Design review of the part shown in the three views and the two pictorial views. Dimensions are in mm from the part's minimum x, y and z. A direction names the side the tool comes from. Coordinates: 2 decimals unless noted, no trailing zeros. Loops run counter-clockwise (first coordinate to the right, second up) from the corner with the lowest first, then second, coordinate; pieces in that order, holes last. Notation, with made-up numbers: M -17,61 L 4,61 A20 ccw 4,75 Z; hole C 43,-27.75 d11. An arc over 180 degrees is marked long. Answer as a JSON object with one key per item and string values. Group by question number.
Item 1: Tool access review of the marked faces 5, 6 and 7: name each direction out of +Z, -Z, +X, -X, +Y, -Y from which nothing blocks a thin tool from reaching the whole face with its end or side.
Item 2: Wall thickness on L1, parallel to Z at x = 24.5, y = 20; L2, parallel to X at y = 10, z = 2.5: over which ranges is each line inside the solid? List them lowest first. Write a range as from..to.
Item 3: Insertion check: pin 1 (4 mm diameter, centred on x = 47.5, z = 11.5, fed in from -Y); pin 2 (7.5 mm diameter, centred on y = 17, z = 30.5, fed in from +X); pin 3 (2 mm diameter, centred on x = 39.5, y = 18, fed in from +Z). Each pin has a flat end and moves straight along its axis. Give the tip position at first contact, or say it passes through.
Item 4: Add section C-C (y = 10.5). State the section outline as (x, z) points, then the cut area to 3 significant figures.
Item 5: Mouldability with a two-part tool opening along Y and no side actions: class the marked faces 1, 2, 3 and 4 as +Y half, -Y half, draft (parallel to the pull), parting line (faces both ways), or undercut.
Item 6: Add section B-B (x = 9.5). State the section outline as (y, z) points.
Item 7: Add section A-A (z = 5). State the section outline as (x, y) points.
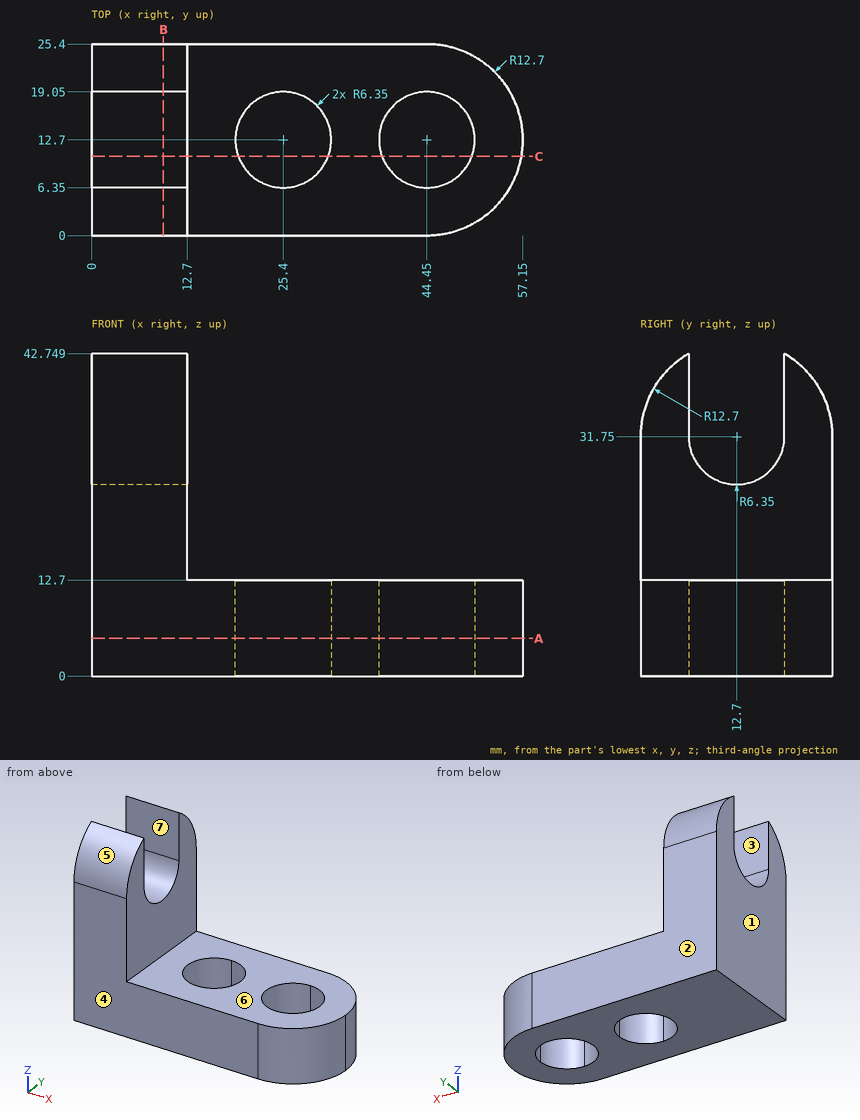
From the geometry:
{
 "1": {"face 5": "+Z, +X, -X, -Y", "face 6": "+Z, +X, +Y, -Y", "face 7": "+Z, +X, -X"},
 "2": {"L1": "z = 0..12.7", "L2": "x = 0..19.65, 31.15..38.7, 50.2..56.86"},
 "3": {"pin 1": "stops at y = 0.04", "pin 2": "stops at x = 12.7", "pin 3": "stops at z = 12.7"},
 "4": {"outline": "M 0,0 L 19.44,0 L 19.44,12.7 L 12.7,12.7 L 12.7,25.79 L 0,25.79 Z; M 31.36,0 L 38.49,0 L 38.49,12.7 L 31.36,12.7 Z; M 50.41,0 L 56.96,0 L 56.96,12.7 L 50.41,12.7 Z", "area": "587 mm²"},
 "5": {"face 1": "draft", "face 2": "+Y half", "face 3": "undercut", "face 4": "-Y half"},
 "6": {"outline": "M 0,0 L 25.4,0 L 25.4,31.75 A12.7 ccw 19.05,42.75 L 19.05,31.75 A6.35 cw 6.35,31.75 L 6.35,42.75 A12.7 ccw 0,31.75 Z"},
 "7": {"outline": "M 0,0 L 44.45,0 A12.7 ccw 44.45,25.4 L 0,25.4 Z; hole C 25.4,12.7 d12.7; hole C 44.45,12.7 d12.7"}
}
